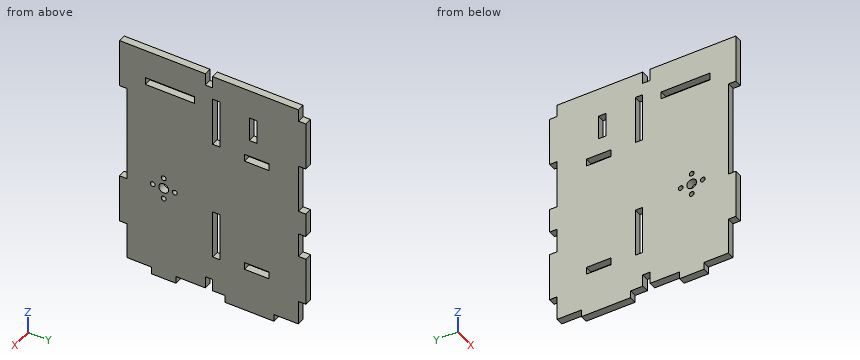
Autodesk Inventor part; units mm, degrees
ref_plane "YZ Plane" through (0, 0, 0) normal (1, 0, 0) x (0, 1, 0)
ref_plane "XZ Plane" through (0, 0, 0) normal (0, 1, 0) x (-1, 0, 0)
ref_plane "XY Plane" through (0, 0, 0) normal (0, 0, 1) x (1, 0, 0)
sketch "Sketch1" plane through (0, 0, 0) normal (1, 0, 0) x (0, 1, 0)
  line L0 (-35, -47.5) -> (35, -47.5)
  line L1 (35, -47.5) -> (35, 47.5)
  line L2 (35, 47.5) -> (-35, 47.5)
  line L3 (-35, 47.5) -> (-35, -47.5)
  line L4 (-35, -47.5) -> (35, 47.5) construction
  line L5 (35, -47.5) -> (-35, 47.5) construction
  point P0 (0, 0)
  dimension "d0" = 70
  dimension "d1" = 95
extrude "Extrusion1" add sketch "Sketch1" along normal blind 3
sketch "Sketch2" plane through (3, 0, 0) normal (1, 0, 0) x (0, 0, -1)
  line L0 (-47.5, -35) -> (47.5, -35)
  line L1 (32.5, -35) -> (12.5, -35)
  line L2 (12.5, -35) -> (12.5, -38)
  line L3 (12.5, -38) -> (32.5, -38)
  line L4 (32.5, -38) -> (32.5, -35)
  line L5 (-27.5, -35) -> (-47.5, -35)
  line L6 (-47.5, -35) -> (-47.5, -38)
  line L7 (-47.5, -38) -> (-27.5, -38)
  line L8 (-27.5, -38) -> (-27.5, -35)
  line L9 (47.5, -35) -> (47.5, 35)
  point P0 (0, 0)
  dimension "d4" = 20
  dimension "d5" = 3
  dimension "d6" = 20
  dimension "d7" = 3
  dimension "d8" = 40
  dimension "d9" = 15
extrude "Extrusion2" add sketch "Sketch2" against normal blind 3
sketch "Sketch3" plane through (3, 0, 0) normal (1, 0, 0) x (0, 0, -1)
  line L0 (47.5, -35) -> (47.5, 35)
  line L1 (47.5, 25) -> (50.5, 25)
  line L2 (50.5, 25) -> (50.5, 5)
  line L3 (50.5, 5) -> (47.5, 5)
  line L4 (47.5, 5) -> (47.5, 25)
  line L5 (47.5, 35) -> (-47.5, 35)
  line L6 (47.5, -15) -> (50.5, -15)
  line L7 (50.5, -15) -> (50.5, -25)
  line L8 (50.5, -25) -> (47.5, -25)
  line L9 (47.5, -25) -> (47.5, -15)
  line L10 (32.5, -35) -> (47.5, -35)
  point P0 (0, 0)
  dimension "d12" = 3
  dimension "d13" = 20
  dimension "d14" = 10
  dimension "d15" = 3
  dimension "d16" = 10
  dimension "d17" = 10
  dimension "d18" = 20
extrude "Extrusion3" add sketch "Sketch3" against normal blind 3
sketch "Sketch4" plane through (3, 0, 0) normal (1, 0, 0) x (0, 0, -1)
  line L0 (32.5, -35) -> (32.5, -38)
  line L1 (40.5, -38) -> (32.5, -38)
  line L2 (40.5, -35) -> (40.5, -38)
  line L3 (32.5, -35) -> (40.5, -35)
  line L4 (12.5, -38) -> (12.5, -35)
  line L5 (-19.5, -35) -> (12.5, -35)
  line L6 (-19.5, -35) -> (-19.5, -38)
  line L7 (12.5, -38) -> (-19.5, -38)
  circle A0 centre (10.5, -20) radius 30 construction
  circle A1 centre (10.5, -20) radius 2
  point P0 (0, 0)
  dimension "d21" = 60
  dimension "d22" = 30
  dimension "d23" = 15
  dimension "d24" = 4
extrude "Extrusion4" cut sketch "Sketch4" against normal blind 3 contours A1
sketch "Sketch5" plane through (3, 0, 0) normal (1, 0, 0) x (0, 0, -1)
  circle A0 centre (10.5, -15.5) radius 1
  circle A1 centre (10.5, -20) radius 2
  circle A2 centre (6, -20) radius 1
  circle A3 centre (10.5, -24.5) radius 1
  circle A4 centre (15, -20) radius 1
  point P0 (0, 0)
  dimension "d27" = 2
  dimension "d28" = 4.5
  dimension "d31" = 360
extrude "Extrusion5" cut sketch "Sketch5" against normal blind 3 contours A0 | A2 | A3 | A4
sketch "Sketch6" plane through (0, 0, 0) normal (-1, 0, 0) x (0, 0, 1)
  line L0 (32.5, -7.5) -> (35.5, -7.5)
  line L1 (35.5, -7.5) -> (35.5, -27.5)
  line L2 (35.5, -27.5) -> (32.5, -27.5)
  line L3 (32.5, -27.5) -> (32.5, -7.5)
  line L4 (-47.5, -15) -> (-47.5, 5)
  line L5 (27.5, -35) -> (-12.5, -35)
  point P0 (0, 0)
  dimension "d35" = 3
  dimension "d36" = 20
  dimension "d37" = 80
  dimension "d38" = 7.5
extrude "Extrusion6" cut sketch "Sketch6" against normal blind 10
sketch "Sketch7" plane through (0, 0, 0) normal (-1, 0, 0) x (0, 0, 1)
  line L0 (-32.5, 3) -> (-12.5, 3)
  line L1 (-12.5, 3) -> (-12.5, 0)
  line L2 (-12.5, 0) -> (-32.5, 0)
  line L3 (-32.5, 0) -> (-32.5, 3)
  line L4 (27.5, -35) -> (-12.5, -35)
  line L5 (-47.5, -15) -> (-47.5, 5)
  line L6 (17.5, 3) -> (37.5, 3)
  line L7 (37.5, 3) -> (37.5, 0)
  line L8 (37.5, 0) -> (17.5, 0)
  line L9 (17.5, 0) -> (17.5, 3)
  point P0 (0, 0)
  dimension "d41" = 20
  dimension "d42" = 3
  dimension "d43" = 35
  dimension "d44" = 15
  dimension "d45" = 20
  dimension "d46" = 3
  dimension "d47" = 30
extrude "Extrusion7" cut sketch "Sketch7" against normal blind 10
sketch "Sketch8" plane through (0, 0, 0) normal (-1, 0, 0) x (0, 0, 1)
  line L0 (-32.5, 23) -> (-29.5, 23)
  line L1 (-29.5, 23) -> (-29.5, 13)
  line L2 (-29.5, 13) -> (-32.5, 13)
  line L3 (-32.5, 13) -> (-32.5, 23)
  line L4 (18.5, 23) -> (15.5, 23)
  line L5 (15.5, 23) -> (15.5, 13)
  line L6 (15.5, 13) -> (18.5, 13)
  line L7 (18.5, 13) -> (18.5, 23)
  line L8 (-47.5, 25) -> (-47.5, 35)
  line L9 (-32.5, 3) -> (-12.5, 3)
  point P0 (0, 0)
  dimension "d50" = 3
  dimension "d51" = 10
  dimension "d52" = 3
  dimension "d53" = 10
  dimension "d54" = 15
  dimension "d55" = 45
  dimension "d56" = 10
extrude "Extrusion8" cut sketch "Sketch8" against normal blind 3
sketch "Sketch9" plane through (3, 0, 0) normal (1, 0, 0) x (0, 0, -1)
  line L0 (-35.5, 18) -> (-25.5, 18)
  line L1 (-25.5, 18) -> (-25.5, 15)
  line L2 (-25.5, 15) -> (-35.5, 15)
  line L3 (-35.5, 15) -> (-35.5, 18)
  line L4 (-37.5, 3) -> (-17.5, 3)
  line L5 (-18.5, 13) -> (-18.5, 23)
  point P0 (0, 0)
  dimension "d59" = 10
  dimension "d60" = 12
  dimension "d61" = 3
  dimension "d62" = 7
extrude "Extrusion9" cut sketch "Sketch9" against normal blind 3
sketch "Sketch10" plane through (0, 0, 0) normal (-1, 0, 0) x (0, 0, 1)
  line L0 (-47.5, 35) -> (47.5, 35)
  line L1 (-37.5, 35) -> (-17.5, 35)
  line L2 (-17.5, 35) -> (-17.5, 38)
  line L3 (-17.5, 38) -> (-37.5, 38)
  line L4 (-37.5, 38) -> (-37.5, 35)
  line L5 (22.5, 35) -> (42.5, 35)
  line L6 (42.5, 35) -> (42.5, 38)
  line L7 (42.5, 38) -> (22.5, 38)
  line L8 (22.5, 38) -> (22.5, 35)
  line L9 (-7.5, 35) -> (2.5, 35)
  line L10 (2.5, 35) -> (2.5, 38)
  line L11 (2.5, 38) -> (-7.5, 38)
  line L12 (-7.5, 38) -> (-7.5, 35)
  line L13 (-47.5, 25) -> (-47.5, 35)
  point P0 (0, 0)
  dimension "d65" = 20
  dimension "d66" = 3
  dimension "d67" = 20
  dimension "d68" = 3
  dimension "d69" = 10
  dimension "d70" = 3
  dimension "d71" = 10
  dimension "d72" = 10
  dimension "d73" = 20
extrude "Extrusion10" add sketch "Sketch10" against normal blind 3
sketch "Sketch11" plane through (0, 0, 0) normal (-1, 0, 0) x (0, 0, 1)
  line L0 (-47.5, -15) -> (-47.5, 5)
  line L1 (-47.5, 0) -> (-42.5, 0)
  line L2 (-42.5, 0) -> (-42.5, -3)
  line L3 (-42.5, -3) -> (-47.5, -3)
  line L4 (-47.5, -3) -> (-47.5, 0)
  line L5 (-12.5, 0) -> (-32.5, 0)
  point P0 (0, 0)
  dimension "d76" = 5
  dimension "d77" = 3
extrude "Extrusion11" cut sketch "Sketch11" against normal blind 3
sketch "Sketch12" plane through (0, 0, 0) normal (-1, 0, 0) x (0, 0, 1)
  line L0 (47.5, 35) -> (47.5, -38)
  line L1 (47.5, 0) -> (42.5, 0)
  line L2 (42.5, 0) -> (42.5, -3)
  line L3 (42.5, -3) -> (47.5, -3)
  line L4 (47.5, -3) -> (47.5, 0)
  line L5 (37.5, 0) -> (17.5, 0)
  point P0 (0, 0)
  dimension "d80" = 3
  dimension "d81" = 5
extrude "Extrusion12" cut sketch "Sketch12" against normal blind 3
properties part number "Motor support"
Source: CAD feature listing. Evaluate the final solid. Frame: model axes, mm. Round coordinates to 2 decimals unless told otherwise and drop trailing zeros. Loops run counter-clockwise (first coordinate to the right, second up) from the corner with the lowest first, then second, coordinate; pieces in that order, holes last. Notation, with made-up numbers: (-38.5, 23) - (-23.5, 23) arc R30 ccw to (-23.5, 49) - close; hole circle Ø5 at (-22.75, -8). An arc over 180 degrees is marked (long way). Write item = value, one per line. Start each with the question number.
Item 1: Section query C-C on z = -15. Output: boundary loops of the cut face in (x, y).
Item 2: Section query B-B on y = -20. Output: boundary loops of the cut face in (x, z).
Item 3: Section query D-D on x = 0.7. Count the separate pieces of the cut face and the enclosed holes in it, plus the area to 3 significant figures.
Item 4: Material intervals for line 1 (Y direction, x = 1, z = -10.5); line 2 (Z direction, x = 1.6, y = 2); line 3 (Z direction, x = 1.6, y = -17.5), sorted ascending.
Item 5: Section query A-A on z = -26. Output: boundary loops of the cut face in (x, y), plus the area to 3 significant figures.
Item 6: First-contact query: pin 1 Ø0.9 at (x, z) = (1, -49.5) entering from +Y; pin 2 Ø1.5 at (x, z) = (1.5, 17) entering from -Y; pin 3 Ø1.2 at (y, z) = (-20, -6) entering from -X; pin 4 Ø0.9 at (x, y) = (1.5, -2) entering from -Z. Flat tips, straight axial feed; report the tip coordinate or a pass-through.
Results list:
q1.outline = (0, -38) - (3, -38) - (3, -21) - (0, -21) - close; (0, -19) - (3, -19) - (3, 0) - (0, 0) - close; (0, 3) - (3, 3) - (3, 35) - (0, 35) - close
q2.outline = (0, -50.5) - (3, -50.5) - (3, -16) - (0, -16) - close; (0, -14) - (3, -14) - (3, -12.5) - (0, -12.5) - close; (0, -8.5) - (3, -8.5) - (3, -7) - (0, -7) - close; (0, -5) - (3, -5) - (3, 32.5) - (0, 32.5) - close; (0, 35.5) - (3, 35.5) - (3, 47.5) - (0, 47.5) - close
q3.separate_pieces = 1
q3.enclosed_holes = 11
q3.area = 6,680 mm²
q4.line_1 = -35 to -25.5, -23.5 to -22, -18 to -16.5, -14.5 to 35
q4.line_2 = -47.5 to -32.5, -12.5 to 17.5, 37.5 to 47.5
q4.line_3 = -50.5 to 32.5, 35.5 to 47.5
q5.outline = (0, -38) - (3, -38) - (3, 0) - (0, 0) - close; (0, 3) - (3, 3) - (3, 38) - (0, 38) - close
q5.area = 219 mm²
q6.pin_1 = 25
q6.pin_2 = -35
q6.pin_3 = through
q6.pin_4 = -42.5
